Can you work these out from the model? Positions are in its coordinate system, mm. Round coordinates to 2 decimals unless told otherwise and drop trailing zeros. Order: outer loops, then holes, each group sorted by start corner. A loop starts at its lowest first (then second) coordinate and runs counter-clockwise, first axis right, second up.
Q1. If we section it at C-C (y = 3): Please give me the cut outline in (x, z), plus the area to 3 significant figures.
Q2. If we section it at A-A (x = 80): Please give me the cut outline in (y, z).
Q3. If we section it at D-D (x = -35.5): Please give me the cut outline in (y, z), plus the area to 3 significant figures.
Q4. Will this pin go through, and if not, where does the flat tip stop? P1, Ø16, axis at x = 80, y = 0, coming from the +Z side.
Q5. If I drill on line 1 (Y direction, x = 80, z = 15.5); line 2 (Y direction, x = -83, z = 6.5), over which ranges is the centre line in solid material (lowest first)?
Q6. We'd pull the mould along Y, two halves only. Please class faces 1 (the face through (-1, 50, 12)), 2 (the face through (-70, 0, 13)), 3 (the face through (2.17, 9.76, 12.67)), 4 (the face through (-1, -50, 12)): pulls with the +Y half, pulls with the -Y half, needs draft (parallel to the pull), parting line crosses it, or undercut.
Q7. If we section it at B-B (z = 8.75): Please give me the cut outline in (x, y).
from build123d import *

# Parameters (mm, degrees)
F0_W     = 200
F0_H     = 100
F1_DEPTH = 25
F2_D     = 20
F2_DEPTH = 25


with BuildPart() as f1:
    # F0 (on Top) → F1 (new body)
    with BuildSketch(Plane.XY):
        Rectangle(F0_W, F0_H)
    extrude(amount=F1_DEPTH)

    # F2
    with Locations(Plane(origin=(0, 0, 0), x_dir=(1, 0, 0), z_dir=(0, 0, -1))):
        with Locations((-80, 0), (-40, 0), (0, 0), (40, 0), (80, 0)):
            Hole(F2_D / 2, depth=F2_DEPTH)


solid = f1.part
Solution:
1. outline: (-100, 0) - (-89.54, 0) - (-89.54, 25) - (-100, 25) - close; (-70.46, 0) - (-49.54, 0) - (-49.54, 25) - (-70.46, 25) - close; (-30.46, 0) - (-9.54, 0) - (-9.54, 25) - (-30.46, 25) - close; (9.54, 0) - (30.46, 0) - (30.46, 25) - (9.54, 25) - close; (49.54, 0) - (70.46, 0) - (70.46, 25) - (49.54, 25) - close; (89.54, 0) - (100, 0) - (100, 25) - (89.54, 25) - close
1. area: 2,620 mm2
2. outline: (-50, 0) - (-10, 0) - (-10, 25) - (-50, 25) - close; (10, 0) - (50, 0) - (50, 25) - (10, 25) - close
3. outline: (-50, 0) - (-8.93, 0) - (-8.93, 25) - (-50, 25) - close; (8.93, 0) - (50, 0) - (50, 25) - (8.93, 25) - close
3. area: 2,050 mm2
4. P1: passes through
5. line 1: y = -50 to -10, 10 to 50
5. line 2: y = -50 to -9.54, 9.54 to 50
6. face 1: pulls with the +Y half
6. face 2: undercut
6. face 3: undercut
6. face 4: pulls with the -Y half
7. outline: (-100, -50) - (100, -50) - (100, 50) - (-100, 50) - close; hole circle Ø20 at (-80, 0); hole circle Ø20 at (-40, 0); hole circle Ø20 at (0, 0); hole circle Ø20 at (40, 0); hole circle Ø20 at (80, 0)
